from build123d import *

# Parameters (mm, degrees)
SKETCH1_W                         = 63.5
SKETCH1_H                         = 70.104
BOSS_EXTRUDE1_DEPTH               = 61.976
SKETCH2_R                         = 45.865892013
CUT_EXTRUDE1_DEPTH                = 63.5
FILLET2_R                         = 12.7
SKETCH3_W                         = 28.956
SKETCH3_H                         = 47.389892013
CUT_EXTRUDE2_DEPTH                = 71.104
SKETCH4_R                         = 6.35
CUT_EXTRUDE3_DEPTH                = 17.110107987
CHAMFER1_SIZE                     = 0.254
FILLET4_R                         = 6.35
SKETCH5_R                         = 10.414
CUT_EXTRUDE4_DEPTH                = 10.922
CUT_EXTRUDE5_REACH                = 54.578
SKETCH6_R                         = 6.35
F_3_8_16_TAPPED_HOLE1_D           = 7.9375
F_3_8_16_TAPPED_HOLE1_DEPTH       = 17.272
F_3_8_16_TAPPED_HOLE1_CSINK_D     = 9.525
F_3_8_16_TAPPED_HOLE1_CSINK_ANGLE = 90
SKETCH9_W                         = 30.5
SKETCH9_H                         = 45.865892013
CUT_EXTRUDE6_DEPTH                = 71.1040001


with BuildPart() as part:
    # Sketch1 → Boss-Extrude1 (new body)
    with BuildSketch(Plane(origin=(0, 0, 0), x_dir=(1, 0, 0), z_dir=(0, 1, 0))):
        with Locations((31.75, 35.052)):
            Rectangle(SKETCH1_W, SKETCH1_H)
    extrude(amount=BOSS_EXTRUDE1_DEPTH)

    # Sketch2 → Cut-Extrude1 (cut)
    with BuildSketch(Plane(origin=(63.5, 0, 0), x_dir=(0, 0, -1), z_dir=(1, 0, 0))):
        with Locations((70.104, 61.976)):
            Circle(SKETCH2_R)
    extrude(amount=-CUT_EXTRUDE1_DEPTH, mode=Mode.SUBTRACT)

    # Fillet2
    fillet2_edges = [part.edges().sort_by_distance(p)[0] for p in [
        (31.75, 61.976, -24.238107987),
        (31.75, 61.976, 0),
    ]]
    fillet(fillet2_edges, radius=FILLET2_R)

    # Sketch3 → Cut-Extrude2 (cut, through all)
    with BuildSketch(Plane(origin=(0, 0, -70.104), x_dir=(-1, 0, 0), z_dir=(0, 0, -1))):
        with Locations((-31.75, 39.805053994)):
            Rectangle(SKETCH3_W, SKETCH3_H)
    extrude(amount=-CUT_EXTRUDE2_DEPTH, mode=Mode.SUBTRACT)

    # Sketch4 → Cut-Extrude3 (cut, through all)
    with BuildSketch(Plane(origin=(0, 16.110107987, 0), x_dir=(1, 0, 0), z_dir=(0, 1, 0))):
        with Locations(Location((31.864756847, 57.404, 0), (0, 0, 270))):  # turned: the seam where the file's is
            Circle(SKETCH4_R)
        with Locations(Location((31.864752163, 12.699481562, 0), (0, 0, 270))):  # turned: the seam where the file's is
            Circle(SKETCH4_R)
    extrude(amount=-CUT_EXTRUDE3_DEPTH, mode=Mode.SUBTRACT)

    # Chamfer1
    chamfer1_edges = [part.edges().sort_by_distance(p)[0] for p in [
        (31.864756847, 16.110107987, -63.754),
        (31.864752163, 16.110107987, -19.049481562),
    ]]
    chamfer(chamfer1_edges, length=CHAMFER1_SIZE)

    # Fillet4
    fillet4_edges = [part.edges().sort_by_distance(p)[0] for p in [
        (0, 8.055053993, -70.104),
        (63.5, 8.055053993, -70.104),
    ]]
    fillet(fillet4_edges, radius=FILLET4_R)

    # Sketch5 → Cut-Extrude4 (cut)
    with BuildSketch(Plane.ZY):
        with Locations((-12.7, 49.276)):
            Circle(SKETCH5_R)
    extrude(amount=-CUT_EXTRUDE4_DEPTH, mode=Mode.SUBTRACT)

    # Sketch6 → Cut-Extrude5 (cut, up to next)
    with BuildSketch(Plane.ZY.offset(-10.922), mode=Mode.PRIVATE) as cut_extrude5_sk1:
        with Locations((-12.7, 49.276)):
            Circle(SKETCH6_R)
    cut_extrude5_tool1 = extrude(cut_extrude5_sk1.sketch, amount=-CUT_EXTRUDE5_REACH, mode=Mode.PRIVATE) & part.part
    add(cut_extrude5_tool1.solids().sort_by_distance((10.922, 49.276, -12.7))[0], mode=Mode.SUBTRACT)

    # 3/8-16 Tapped Hole1
    with Locations(Plane(origin=(63.5, 0, 0), x_dir=(0, 0, -1), z_dir=(1, 0, 0))):
        with Locations((12.7, 49.276)):
            CounterSinkHole(F_3_8_16_TAPPED_HOLE1_D / 2, F_3_8_16_TAPPED_HOLE1_CSINK_D / 2, depth=F_3_8_16_TAPPED_HOLE1_DEPTH, counter_sink_angle=F_3_8_16_TAPPED_HOLE1_CSINK_ANGLE)

    # Sketch9 → Cut-Extrude6 (cut, through all)
    with BuildSketch(Plane.XY):
        with Locations((31.75, 39.043053994)):
            Rectangle(SKETCH9_W, SKETCH9_H)
    extrude(amount=-CUT_EXTRUDE6_DEPTH, mode=Mode.SUBTRACT)


solid = part.part
Read the model definition and answer for the solid it produces. Units are mm, in the model's axes. A direction names the side the tool comes from. Coordinates: 2 decimals unless noted, no trailing zeros. Order: outer loops, then holes, each group sorted by start corner. A loop starts at its lowest first (then second) coordinate and runs counter-clockwise, first axis right, second up. Notation, with made-up numbers: (68.25, 50.25) - (95.25, 50.25) arc R13 cw to (95.25, 62.25) - close; hole circle Ø1 at (36, 85.25). An arc over 180 degrees is marked (long way). Use one line per item in the form item = value.
(1) Section D-D, the plane x = 14.5 is taken. Give the vertices of the cut face in (y, z), then the cut area to 3 significant figures.
Computed values:
outline = (0, -70.1) - (16.11, -70.1) arc R45.87 cw to (52.03, -25.33) arc R12.7 ccw to (61.98, -12.93) - (61.98, -12.7) arc R12.7 ccw to (49.28, 0) - (0, 0) - close; hole circle Ø12.7 at (49.28, -12.7)
area = 2,510 mm²
(2) Given pin 1 Ø15 at (x, z) = (28, -40.5) entering from +Y; pin 2 Ø2 at (x, y) = (55, 37) entering from -Z; pin 3 Ø3 at (x, y) = (16.5, 29) entering from -Z; pin 4 Ø24 at (y, z) = (49.276, -12.7) entering from -X, each flat-ended and moving along its own axis, determine where each tip first touches the part or whether it passes through.
Computed values:
pin_1 = 16.11
pin_2 = -32.3
pin_3 = -39.85
pin_4 = 0
(3) For a pull along Y with two mould halves and no side action, classify faces 3 (the face through (54.74, 53.21, -13.22)), 4 (the face through (55.37, 59.11, -20.97)), 5 (the face through (63.5, 24, -24)), 6 (the face through (10.922, 54, -8)) as pulls with the +Y half, pulls with the -Y half, needs draft (parallel to the pull), parting line crosses it, or undercut.
Computed values:
face_3 = undercut
face_4 = pulls with the +Y half
face_5 = needs draft
face_6 = undercut
(4) Section B-B, the plane y = 32 is taken. Give the vertices of the cut face in (x, z), then the cut area to 3 significant figures.
Computed values:
outline = (0, -35.39) - (16.5, -35.39) - (16.5, 0) - (0, 0) - close; (47, -35.39) - (63.5, -35.39) - (63.5, 0) - (47, 0) - close
area = 1,170 mm²
(5) Section A-A, the plane x = 50 is taken. Give the vertices of the cut face in (y, z).
Computed values:
outline = (0, -70.1) - (16.11, -70.1) arc R45.87 cw to (52.03, -25.33) arc R12.7 ccw to (61.98, -12.93) - (61.98, -12.7) arc R12.7 ccw to (49.28, 0) - (0, 0) - close; hole circle Ø7.94 at (49.28, -12.7)
(6) Which of the six approach directions +Z, -Z, +X, -X, +Y, -Y give full straight-line access (tool end or side, diameter ignored) to faces 1 (the face through (47, 34, -19)), 2 (the face through (28, 8.04, -62.44))?
Computed values:
face_1 = +Z, -Z, +Y
face_2 = +Y, -Y
(7) Straight lines are drawn through the part: L1, parallel to X at y = 40, z = -23; L2, parallel to X at y = 47.5, z = -19.5; L3, parallel to Y at x = 45, z = -8. For each, find the intervals that lie inside material, in ascending order.
Computed values:
L1 = 0 to 16.5, 47 to 63.5
L2 = 10.92 to 16.5, 47 to 63.5
L3 = 0 to 16.11
(8) Section C-C, the plane y = 7.5 is taken. Give the vertices of the cut face in (x, z), then the cut area to 3 significant figures.
Computed values:
outline = (0, -63.75) arc R6.35 ccw to (6.35, -70.1) - (57.15, -70.1) arc R6.35 ccw to (63.5, -63.75) - (63.5, 0) - (0, 0) - close; hole circle Ø12.7 at (31.86, -57.4); hole circle Ø12.7 at (31.86, -12.7)
area = 4,180 mm²
